```python
from build123d import *

# Parameters (mm, degrees)
SKETCH_1_R          = 3.5
EXTRUDE_1_DEPTH     = 140
SKETCH_2_W          = 31.2
SKETCH_2_H          = 17.479956732
CUT_EXTRUDE_1_DEPTH = 50
CUT_EXTRUDE_2_DEPTH = 60
SKETCH_4_R          = 3.2
CUT_EXTRUDE_3_DEPTH = 140.649970789
SKETCH_5_W          = 88.266499161
SKETCH_5_H          = 80
CUT_EXTRUDE_4_DEPTH = 165.458365818


with BuildPart() as part:
    # 草图1 → 凸台-拉伸1 (new body)
    with BuildSketch(Plane.XY):
        with BuildLine():
            Line((-77.479727509, -5.387494924), (75.786771652, -5.387494924))
            ThreePointArc((75.786771652, -5.387494924), (79.659754999, 8.535121366), (69.153522072, -1.387494924))
            Line((69.153522072, -1.387494924), (-70.846477928, -1.387494924))
            ThreePointArc((-70.846477928, -1.387494924), (-81.352710855, 8.535121366), (-77.479727509, -5.387494924))
        make_face()
        with Locations((-77.479727509, 2.112505076)):
            Circle(SKETCH_1_R, mode=Mode.SUBTRACT)
        Polygon((77.386771652, 4.883786368), (74.186771652, 4.883786368), (72.586771652, 2.112505076), (74.186771652, -0.658776216), (77.386771652, -0.658776216), (78.986771652, 2.112505076), align=None, mode=Mode.SUBTRACT)
    extrude(amount=-EXTRUDE_1_DEPTH)

    # 草图2 → 切除-拉伸1 (cut)
    with BuildSketch(Plane(origin=(-69.979727509, 0, 0), x_dir=(0, 0, -1), z_dir=(1, 0, 0))):
        with Locations((15.6, 0.87252671)):
            Rectangle(SKETCH_2_W, SKETCH_2_H)
        with Locations((124.4, 0.87252671)):
            Rectangle(SKETCH_2_W, SKETCH_2_H)
    extrude(amount=-CUT_EXTRUDE_1_DEPTH, mode=Mode.SUBTRACT)

    # 草图3 → 切除-拉伸2 (cut)
    with BuildSketch(Plane.ZY.offset(-68.286771652)):
        Polygon((-109.6, -19.072953763), (-30.4, -19.072953763), (-29.6, -19.072953763), (-29.6, 22.402056511), (-29.61, 22.402056511), (-110.39, 22.402056511), (-110.4, 22.402056511), (-110.4, -19.072953763), align=None)
    extrude(amount=-CUT_EXTRUDE_2_DEPTH, mode=Mode.SUBTRACT)

    # 草图4 → 切除-拉伸3 (cut, through all)
    with BuildSketch(Plane(origin=(0, 0, -29.6), x_dir=(-1, 0, 0), z_dir=(0, 0, -1))):
        with Locations((-75.786771652, 2.112505076)):
            Circle(SKETCH_4_R)
    extrude(amount=-CUT_EXTRUDE_3_DEPTH, mode=Mode.SUBTRACT)

    # 草图5 → 切除-拉伸4 (cut, through all)
    with BuildSketch(Plane.XZ.offset(5.387494924)):
        with Locations((-0.846477928, -70)):
            Rectangle(SKETCH_5_W, SKETCH_5_H)
    extrude(amount=-CUT_EXTRUDE_4_DEPTH, mode=Mode.SUBTRACT)


solid = part.part
```
The listing builds one solid part. Answer for the finished solid, in the listing's coordinates (mm). A direction names the side the tool comes from. Coordinates: 2 decimals unless noted, no trailing zeros. Order: outer loops, then holes, each group sorted by start corner. A loop starts at its lowest first (then second) coordinate and runs counter-clockwise, first axis right, second up. Notation, with made-up numbers: M 68.5,-5.75 L 87.5,-5.75 A38 ccw 87.5,33.25 Z; hole C 56.25,65 d7. An arc over 180 degrees is marked long. Answer as a JSON object with one key per item and string values. Group by question number.
1. Section A-A on z = -94 is taken. Write down the section's boundary in (x, y).
2. Section C-C on x = 40 is taken. Write down the section's boundary in (y, z).
3. Section D-D on x = -56.5 is taken. Write down the section's boundary in (y, z), then the cut area to 3 significant figures.
4. Flat-ended cylindrical pins translate along their axes: P1, Ø3, axis at y = -3.5, z = -12.5, coming from the -X side; P2, Ø2, axis at y = -2.5, z = -64.5, coming from the -X side; P3, Ø4.5, axis at x = -76.5, y = 1.5, coming from the -Z side; P4, Ø9, axis at x = -77.48, y = 2.11, coming from the -Z side. Find the tip coordinate at first contact, or state that the pin passes through.
5. Section B-B on z = -129 is taken. Write down the section's boundary in (x, y), then the cut area to 3 significant figures.
6. Straight lines are drawn through the part: line 1 (X direction, y = 1.75, z = -6.5); line 2 (X direction, y = 2, z = -59.5); line 3 (Z direction, x = -31.5, y = -3). For each, find the intervals that lie inside material, in ascending order.
7. Determine the mould class of faces 6 (the flat face through (43.287, -3, -71)), 7 (the cylindrical face through (-74.247, 0.772, -69.457)), 8 (the flat face through (-75.7, -1.3, -31.2)) for opening direction Z: released by +Z, released by -Z, zero draft, split by the parting line, or undercut.
8. A tool of negligible diameter and unlimited length cuts with its end or side. For faces 1 (the cylindrical face through (72.735, 3.074, -15.007)), 2 (the flat face through (-69.98, -3, -15)), 3 (the flat face through (75.7, -1.3, -29.6)), 4 (the flat face through (-75.7, -1.3, -108.8)), 5 (the flat face through (-1, -3, -30)), from which of +Z, -Z, +X, -X, +Y, -Y can it reach the whole face along a straight path? Write none if from no direction.
Values follow:
{
 "1": {"outline": "M -77.48,-5.39 L -44.98,-5.39 L -44.98,-1.39 L -70.85,-1.39 A7.5 ccw long Z; M 43.29,-5.39 L 68.29,-5.39 L 68.29,-1.39 L 43.29,-1.39 Z; hole C -77.48,2.11 d7"},
 "2": {"outline": "M -5.39,-140 L -1.39,-140 L -1.39,-110 L -5.39,-110 Z; M -5.39,-30 L -1.39,-30 L -1.39,0 L -5.39,0 Z"},
 "3": {"outline": "M -5.39,-140 L -1.39,-140 L -1.39,0 L -5.39,0 Z", "area": "560 mm2"},
 "4": {"P1": "x = -69.98", "P2": "x = -84.05", "P3": "through", "P4": "z = -108.8"},
 "5": {"outline": "M -69.98,-5.39 L 75.79,-5.39 A7.5 ccw long 69.15,-1.39 L -69.98,-1.39 Z; hole M 72.59,2.11 L 74.19,-0.66 L 77.39,-0.66 L 78.99,2.11 L 77.39,4.88 L 74.19,4.88 Z", "area": "714 mm2"},
 "6": {"line 1": "68.3 to 72.61, 78.97 to 83.28", "line 2": "-84.98 to -80.98, -73.98 to -69.98", "line 3": "-140 to -110, -30 to 0"},
 "7": {"face 6": "undercut", "face 7": "zero draft", "face 8": "released by +Z"},
 "8": {"face 1": "+Z", "face 2": "+Z, -X, +Y, -Y", "face 3": "+X, +Y, -Y", "face 4": "-Z, -X, +Y, -Y", "face 5": "+Y, -Y"}
}
